Geometry: final body of the model. Coordinates: model frame, mm. A direction names the side the tool comes from. Coordinates: 2 decimals unless noted, no trailing zeros. Write item = value, one per line.
from build123d import *

# Parameters (mm, degrees)
BOSS_EXTRU_1_DEPTH      = 5
ESQUISSE2_R             = 1.5
ENL_V_MAT_EXTRU_1_DEPTH = 209.56953277
ESQUISSE4_R             = 1.25
ENL_V_MAT_EXTRU_3_DEPTH = 209.56953277
ESQUISSE5_R             = 1.5
ENL_V_MAT_EXTRU_6_DEPTH = 269.378676152


with BuildPart() as part:
    # Esquisse1 → Boss.-Extru.1 (new body)
    with BuildSketch(Plane(origin=(0, 0, 0), x_dir=(1, 0, 0), z_dir=(0, 1, 0))):
        with BuildLine():
            Line((123.5, -119.464880645), (123.5, 36.2))
            Line((123.5, 36.2), (-123.5, 36.2))
            Line((-123.5, 36.2), (-123.5, -119.464880645))
            Line((-123.5, -119.464880645), (-118.5, -119.464880645))
            ThreePointArc((-118.5, -119.464880645), (-104.357864376, -125.322745021), (-98.5, -139.464880645))
            Line((-98.5, -139.464880645), (-98.5, -168))
            Line((-98.5, -168), (98.5, -168))
            Line((98.5, -168), (98.5, -139.464880645))
            ThreePointArc((98.5, -139.464880645), (104.357864376, -125.322745021), (118.5, -119.464880645))
            Line((118.5, -119.464880645), (123.5, -119.464880645))
        make_face()
    extrude(amount=-BOSS_EXTRU_1_DEPTH)

    # Esquisse2 → Enlèv. mat.-Extru.1 (cut, through all)
    with BuildSketch(Plane(origin=(0, 0, 0), x_dir=(1, 0, 0), z_dir=(0, 1, 0))):
        with Locations(Location((-118.5, 11.2, 0), (0, 0, 270))):
            Circle(ESQUISSE2_R)
        with Locations(Location((118.5, 11.2, 0), (0, 0, 270))):
            Circle(ESQUISSE2_R)
    extrude(amount=-ENL_V_MAT_EXTRU_1_DEPTH, mode=Mode.SUBTRACT)

    # Esquisse4 → Enlèv. mat.-Extru.3 (cut, through all)
    with BuildSketch(Plane(origin=(0, 0, 0), x_dir=(1, 0, 0), z_dir=(0, 1, 0))):
        with Locations(Location((0, -129.5, 0), (0, 0, 270))):
            Circle(ESQUISSE4_R)
        with Locations(Location((29.5, -100, 0), (0, 0, 270))):
            Circle(ESQUISSE4_R)
        with Locations(Location((-29.5, -100, 0), (0, 0, 270))):
            Circle(ESQUISSE4_R)
        with Locations(Location((0, -70.5, 0), (0, 0, 270))):
            Circle(ESQUISSE4_R)
    extrude(amount=-ENL_V_MAT_EXTRU_3_DEPTH, mode=Mode.SUBTRACT)

    # Esquisse5 → Enlèv. mat.-Extru.6 (cut, through all)
    with BuildSketch(Plane(origin=(0, -179.424124514, 11.214007782), x_dir=(1, 0, 0), z_dir=(0, 0.9980525784828886, -0.06237828615518076))):
        with Locations(Location((-17.5, -104.583435434, 0), (0, 0, 270))):
            Circle(ESQUISSE5_R)
        with Locations(Location((-25, -96.451522388, 0), (0, 0, 270))):
            Circle(ESQUISSE5_R)
        with Locations(Location((-82.5, -104.583435434, 0), (0, 0, 270))):
            Circle(ESQUISSE5_R)
        with Locations(Location((-75, -96.451522388, 0), (0, 0, 270))):
            Circle(ESQUISSE5_R)
        with Locations(Location((17.5, -104.583435434, 0), (0, 0, 270))):
            Circle(ESQUISSE5_R)
        with Locations(Location((25, -96.451522388, 0), (0, 0, 270))):
            Circle(ESQUISSE5_R)
        with Locations(Location((75, -96.451522388, 0), (0, 0, 270))):
            Circle(ESQUISSE5_R)
        with Locations(Location((82.5, -104.583435434, 0), (0, 0, 270))):
            Circle(ESQUISSE5_R)
    extrude(amount=ENL_V_MAT_EXTRU_6_DEPTH, mode=Mode.SUBTRACT)


solid = part.part
1) Pin query (flat end, axial travel): pin 1 (1 mm diameter, centred on x = 95, z = -1, fed in from +Y); pin 2 (3 mm diameter, centred on y = -1, z = 129, fed in from -X); pin 3 (2 mm diameter, centred on x = 0, z = 70.5, fed in from +Y); pin 4 (2.5 mm diameter, centred on y = -1.5, z = 151.5, fed in from +X). Return the tip coordinate at first contact, or that it passes through.
Numbers:
pin_1 = 0
pin_2 = -102.47
pin_3 = through
pin_4 = 98.5
2) Section A-A, the plane y = -3.4. Give the number of separate pieces and of enclosed holes in the cut face, and give its area (3 significant figures).
Numbers:
separate_pieces = 1
enclosed_holes = 14
area = 48,100 mm²
3) Set-up query: faces 1 (the face through (-121, -2, 119.465)), 2 (the face through (121, -2, 119.465)), 3 (the face through (123.5, -2, 43)). Return all of +Z, -Z, +X, -X, +Y, -Y with unobstructed straight access to the full face (end or side cutting, diameter ignored); none if empty.
Numbers:
face_1 = +Z, -X, +Y, -Y
face_2 = +Z, +X, +Y, -Y
face_3 = +Z, -Z, +X, +Y, -Y
4) Line query: L1, parallel to X at y = -1.55, z = -11.2; L2, parallel to X at y = -1.3, z = 70.5; L3, parallel to Z at x = -118.5, y = -1.8. Output: solid intervals per line, ascending.
Numbers:
L1 = -123.5 to -120, -117 to 117, 120 to 123.5
L2 = -123.5 to -1.25, 1.25 to 123.5
L3 = -36.2 to -12.7, -9.7 to 119.46
